The model under review builds one solid part; all positions refer to its coordinate system, in mm. Coordinates: 2 decimals unless noted, no trailing zeros. Write each loop counter-clockwise with the first axis right and the second up, starting at its lowest first coordinate (ties: lowest second). Pieces come first, ordered by that corner, then holes.
1) Add section B-B, the plane y = -1.5. State the section outline as (x, z) points.
2) For P1, Ø4.5, axis at x = 16.8, y = -6.5, coming from the +Z side, flat-tipped, find the tip position at first contact; note if it passes through.
3) Add section C-C, the plane z = 1.7. State the section outline as (x, y) points.
4) Add section A-A, the plane x = -3. State the section outline as (y, z) points.
5) For line 1 (Y direction, x = -3, z = 0.35); line 2 (X direction, y = 12.5, z = 0.2); line 3 (X direction, y = -1.5, z = 0.3), list the stretches that pass through material, from the lowest coordinate up.
6) Add section D-D, the plane y = 12.5. State the section outline as (x, z) points, then the cut area to 3 significant figures.
7) Mouldability with a two-part tool opening along Y and no side actions: class faces 1 (the cylindrical face through (18.46, -6.13, 0.28)), 2 (the flat face through (0, -17.5, 1)), 3 (the flat face through (0, 17.5, 1)) as released by +Y, released by -Y, zero draft, split by the parting line, or undercut.
from build123d import *

# Parameters (mm, degrees)
SKETCH1_W                                    = 58
SKETCH1_H                                    = 35
BOSS_EXTRUDE1_DEPTH                          = 2
CSK_FOR_M3_FLAT_COUNTERSUNK_HEAD_SCR_2_COUNT = 2
CSK_FOR_M3_FLAT_COUNTERSUNK_HEAD_SCR_2_PITCH = 20
CSK_FOR_M3_FLAT_COUNTERSUNK_HEAD_SCR_3_COUNT = 2
CSK_FOR_M3_FLAT_COUNTERSUNK_HEAD_SCR_3_PITCH = 39.8
CSK_FOR_M3_FLAT_COUNTERSUNK_HEAD_SCR_4_COUNT = 2
CSK_FOR_M3_FLAT_COUNTERSUNK_HEAD_SCR_4_PITCH = 44.102607633
CSK_FOR_M3_FLAT_COUNTERSUNK_HEAD_SCR_5_COUNT = 2
CSK_FOR_M3_FLAT_COUNTERSUNK_HEAD_SCR_5_PITCH = 14


with BuildPart() as part:
    # Sketch1 → Boss-Extrude1 (new body)
    with BuildSketch(Plane.XY):
        Rectangle(SKETCH1_W, SKETCH1_H)
    extrude(amount=BOSS_EXTRUDE1_DEPTH)

    # Sketch3 → CSK for M3 Flat Countersunk Head Screw1 (revolve, cut)
    with BuildSketch(Plane(origin=(-23, 12.5, 2), x_dir=(0, -1, 0), z_dir=(1, 0, 0))):
        Polygon((0, 0), (0, 2), (1.7, 2), (1.7, 1.45), (3.15, 0), align=None)
    csk_for_m3_flat_countersunk_head_screw1 = revolve(axis=Axis((-23, 12.5, 8.35), (0, 0, -1)), mode=Mode.SUBTRACT)

    # CSK for M3 Flat Countersunk Head Scr 2: CSK for M3 Flat Countersunk Head Screw1 ×2
    with Locations(*[(i * CSK_FOR_M3_FLAT_COUNTERSUNK_HEAD_SCR_2_PITCH, 0, 0) for i in range(1, CSK_FOR_M3_FLAT_COUNTERSUNK_HEAD_SCR_2_COUNT)]):
        add(csk_for_m3_flat_countersunk_head_screw1, mode=Mode.SUBTRACT)

    # CSK for M3 Flat Countersunk Head Scr 3: CSK for M3 Flat Countersunk Head Screw1 ×2
    with Locations(*[(i * CSK_FOR_M3_FLAT_COUNTERSUNK_HEAD_SCR_3_PITCH, 0, 0) for i in range(1, CSK_FOR_M3_FLAT_COUNTERSUNK_HEAD_SCR_3_COUNT)]):
        add(csk_for_m3_flat_countersunk_head_screw1, mode=Mode.SUBTRACT)

    # CSK for M3 Flat Countersunk Head Scr 4: CSK for M3 Flat Countersunk Head Screw1 ×2
    with Locations(*[Vector(0.90244097, -0.430813528, 0) * (i * CSK_FOR_M3_FLAT_COUNTERSUNK_HEAD_SCR_4_PITCH) for i in range(1, CSK_FOR_M3_FLAT_COUNTERSUNK_HEAD_SCR_4_COUNT)]):
        add(csk_for_m3_flat_countersunk_head_screw1, mode=Mode.SUBTRACT)

    # CSK for M3 Flat Countersunk Head Scr 5: CSK for M3 Flat Countersunk Head Screw1 ×2
    with Locations(*[(0, -i * CSK_FOR_M3_FLAT_COUNTERSUNK_HEAD_SCR_5_PITCH, 0) for i in range(1, CSK_FOR_M3_FLAT_COUNTERSUNK_HEAD_SCR_5_COUNT)]):
        add(csk_for_m3_flat_countersunk_head_screw1, mode=Mode.SUBTRACT)


solid = part.part
Geometry results:
1. outline: (-29, 0) - (-24.7, 0) - (-24.7, 0.55) - (-26.15, 2) - (-29, 2) - close; (-21.3, 0) - (29, 0) - (29, 2) - (-19.85, 2) - (-21.3, 0.55) - close
2. P1: stops at z = 1.1
3. outline: (-29, -17.5) - (29, -17.5) - (29, 17.5) - (-29, 17.5) - close; hole circle Ø5.7 at (-23, -1.5); hole circle Ø5.7 at (-23, 12.5); hole circle Ø5.7 at (-3, 12.5); hole circle Ø5.7 at (16.8, -6.5); hole circle Ø5.7 at (16.8, 12.5)
4. outline: (-17.5, 0) - (10.8, 0) - (10.8, 0.55) - (9.35, 2) - (-17.5, 2) - close; (14.2, 0) - (17.5, 0) - (17.5, 2) - (15.65, 2) - (14.2, 0.55) - close
5. line 1: y = -17.5 to 10.8, 14.2 to 17.5
5. line 2: x = -29 to -24.7, -21.3 to -4.7, -1.3 to 15.1, 18.5 to 29
5. line 3: x = -29 to -24.7, -21.3 to 29
6. outline: (-29, 0) - (-24.7, 0) - (-24.7, 0.55) - (-26.15, 2) - (-29, 2) - close; (-21.3, 0) - (-4.7, 0) - (-4.7, 0.55) - (-6.15, 2) - (-19.85, 2) - (-21.3, 0.55) - close; (-1.3, 0) - (15.1, 0) - (15.1, 0.55) - (13.65, 2) - (0.15, 2) - (-1.3, 0.55) - close; (18.5, 0) - (29, 0) - (29, 2) - (19.95, 2) - (18.5, 0.55) - close
6. area: 89.3 mm2
7. face 1: undercut
7. face 2: released by -Y
7. face 3: released by +Y
